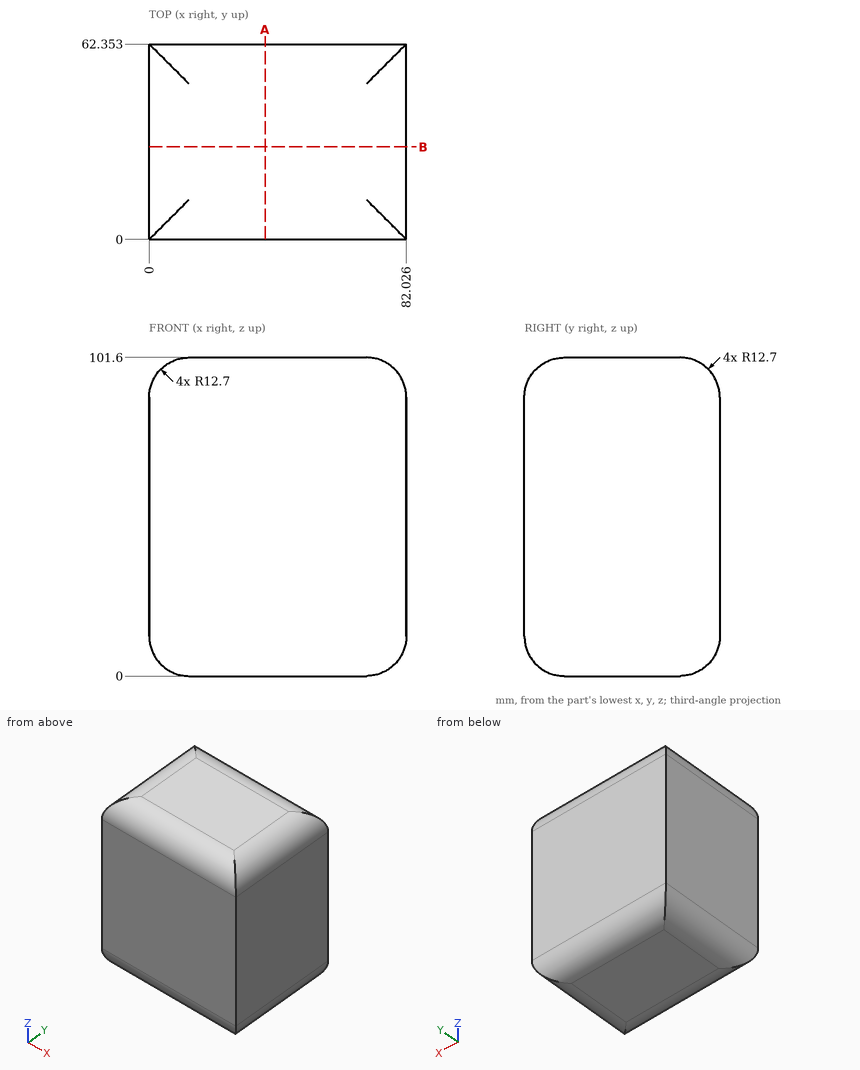
Verification items for this drawing (mm, ordinates from the low corner). Coordinates: 2 decimals unless noted, no trailing zeros. Order: outer loops, then holes, each group sorted by start corner. A loop starts at its lowest first (then second) coordinate and runs counter-clockwise, first axis right, second up. Notation, with made-up numbers: M 9,-21 L 56,-21 A33 ccw 56,13 Z; hole C -28,-4.75 d6. An arc over 180 degrees is marked long. One line per item, written item: value. Start each with the question number.
Item 1: Sectioned sample at B-B on y = 29.5. Record the cut outline in (x, z).
Item 2: Thickness scan on probe 1 along Y at (x, z) = (9.5, 12.5); probe 2 along Z at (x, y) = (35, 10); probe 3 along Z at (x, y) = (69, 56). Record the ranges inside material, lowest first.
Item 3: Sectioned sample at A-A on x = 37. Record the cut outline in (y, z), then the cut area to 3 significant figures.
Item 4: Depth check by flat-ended pin: P1, Ø1.5, axis at y = 13, z = 10, coming from the -X side; P2, Ø1, axis at x = 14.5, y = 10, coming from the -Z side. Enter the tip coordinate at first touch or a pass-through.
Calculated:
1. outline: M 0,12.7 A12.7 ccw 12.7,0 L 69.33,0 A12.7 ccw 82.03,12.7 L 82.03,88.9 A12.7 ccw 69.33,101.6 L 12.7,101.6 A12.7 ccw 0,88.9 Z
2. probe 1: 0 to 62.35
2. probe 2: 0.29 to 101.31
2. probe 3: 1.7 to 99.9
3. outline: M 0,12.7 A12.7 ccw 12.7,0 L 49.65,0 A12.7 ccw 62.35,12.7 L 62.35,88.9 A12.7 ccw 49.65,101.6 L 12.7,101.6 A12.7 ccw 0,88.9 Z
3. area: 6,200 mm^2
4. P1: x = 0.15
4. P2: z = 0.19
